from build123d import *

# Parameters (mm, degrees)
F1_DEPTH = 9
F2_DEPTH = 4.6
F3_SIZE  = 1


with BuildPart() as f1:
    # F0 (on Top) → F1 (new body)
    with BuildSketch(Plane.XY):
        with BuildLine():
            ThreePointArc((4.4395945761, 2.3), (-5, 0), (4.4395945761, -2.3))
            Line((4.4395945761, -2.3), (2.2961925006, -2.3))
            ThreePointArc((2.2961925006, -2.3), (-3.25, 0), (2.2961925006, 2.3))
            Line((2.2961925006, 2.3), (4.4395945761, 2.3))
        make_face()
        with BuildLine():
            Line((2.2961925006, -2.3), (4.4395945761, -2.3))
            ThreePointArc((4.4395945761, -2.3), (4.8578788005, -1.1836441863), (5, 0))
            ThreePointArc((5, 0), (4.8578788005, 1.1836441863), (4.4395945761, 2.3))
            Line((4.4395945761, 2.3), (2.2961925006, 2.3))
            ThreePointArc((2.2961925006, 2.3), (3.0020930721, 1.244964733), (3.25, 0))
            ThreePointArc((3.25, 0), (3.0020930721, -1.244964733), (2.2961925006, -2.3))
        make_face()
    extrude(amount=F1_DEPTH)

    # F0 (on Top) → F2 (join)
    with BuildSketch(Plane.XY):
        with BuildLine():
            Line((4.4395945761, -2.3), (9.6, -2.3))
            Line((9.6, -2.3), (9.6, 2.3))
            Line((9.6, 2.3), (4.4395945761, 2.3))
            ThreePointArc((4.4395945761, 2.3), (4.8578788005, 1.1836441863), (5, 0))
            ThreePointArc((5, 0), (4.8578788005, -1.1836441863), (4.4395945761, -2.3))
        make_face()
    extrude(amount=F2_DEPTH)

    # F3
    f3_edges = [f1.edges().sort_by_distance(p)[0] for p in [
        (9.6, -2.3, 2.3),
        (9.6, 2.3, 2.3),
    ]]
    chamfer(f3_edges, length=F3_SIZE)


solid = f1.part
Design review of the part built by this model. Coordinates are the model's own, in mm. A direction names the side the tool comes from. Give positions to 0.01 mm unless a question says otherwise; leave off trailing zeros. Write each loop counter-clockwise with the first axis right and the second up, starting at its lowest first coordinate (ties: lowest second). Pieces come first, ordered by that corner, then holes. Notation, with made-up numbers: M 45,-34 L 65,-34 A21 cw 65,-29 Z; hole C 54,71.25 d1. An arc over 180 degrees is marked long. Return JSON: item names as keys, results as strings. Group by question number.
Item 1: Take a section at B-B (z = 2.5). Give the boundary of the cut face in (x, y).
Item 2: Tool access review of faces 1 (the flat face through (6, -2.3, 2)), 2 (the flat face through (9.6, 0, 2)), 3 (the flat face through (7, 2.3, 2)): name each direction out of +Z, -Z, +X, -X, +Y, -Y from which nothing blocks a thin tool from reaching the whole face with its end or side.
Item 3: Take a section at C-C (y = -0.75). Give the boundary of the cut face in (x, z).
Item 4: Take a section at A-A (x = 0). Give the boundary of the cut face in (y, z), plus the area to 3 significant figures.
Item 5: Wall thickness on line 1 along Y through (x, z) = (0, 2.5); line 2 along X through (y, z) = (-3, 4.75); line 3 along Y through (x, z) = (6, 0.75): over which ranges is each line inside the solid? List them lowest first.
Item 6: Take a section at D-D (x = 8). Give the boundary of the cut face in (y, z), plus the area to 3 significant figures.
Item 7: Clearance check with flat-ended pins moving along their axes: pin 1 Ø1 at (x, z) = (4, 2.5) entering from +Y; pin 2 Ø4.5 at (x, z) = (7.5, 3) entering from +Y; pin 3 Ø4.5 at (x, z) = (6.5, 3.5) entering from -Y. State where each tip first meets the part, or that it passes through.
Return value:
{
 "1": {"outline": "M 4.44,-2.3 L 8.6,-2.3 L 9.6,-1.3 L 9.6,1.3 L 8.6,2.3 L 4.44,2.3 A5 ccw long Z; hole C 0,0 d6.5"},
 "2": {"face 1": "+Z, -Z, +X, -Y", "face 2": "+Z, -Z, +X, +Y, -Y", "face 3": "+Z, -Z, +X, +Y"},
 "3": {"outline": "M -4.94,0 L -3.16,0 L -3.16,9 L -4.94,9 Z; M 3.16,0 L 9.6,0 L 9.6,4.6 L 4.94,4.6 L 4.94,9 L 3.16,9 Z"},
 "4": {"outline": "M -5,0 L -3.25,0 L -3.25,9 L -5,9 Z; M 3.25,0 L 5,0 L 5,9 L 3.25,9 Z", "area": "31.5 mm2"},
 "5": {"line 1": "y = -5 to -3.25, 3.25 to 5", "line 2": "x = -4 to -1.25, 1.25 to 4", "line 3": "y = -2.3 to 2.3"},
 "6": {"outline": "M -2.3,0 L 2.3,0 L 2.3,4.6 L -2.3,4.6 Z", "area": "21.2 mm2"},
 "7": {"pin 1": "stops at y = 3.57", "pin 2": "stops at y = 2.3", "pin 3": "stops at y = -2.63"}
}
